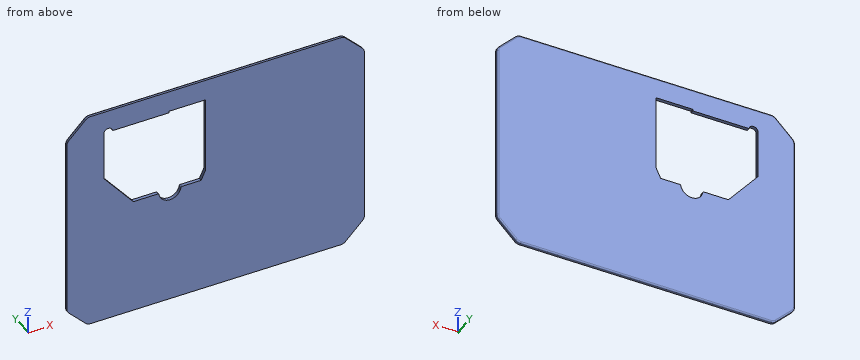
from build123d import *

# Parameters (mm, degrees)
BOSS_EXTRUDE1_DEPTH = 2.5
FILLET2_R           = 5
FILLET3_R           = 1


with BuildPart() as part:
    # Sketch1 → Boss-Extrude1 (new body)
    with BuildSketch(Plane(origin=(0, 0, 0), x_dir=(1, 0, 0), z_dir=(0, 1, 0))):
        Polygon((137.875, 109.125), (-52.875, 109.125), (-68.375, 93.625), (-68.375, -43.375), (-52.875, -58.875), (137.875, -58.875), (153.375, -43.375), (153.375, 93.625), align=None)
        with BuildLine():
            Line((-40.875, -5.193242225), (-18.827366795, 21.125))
            Line((-18.827366795, 21.125), (0.240165454, 21.125))
            ThreePointArc((0.240165454, 21.125), (8.475, 28.875), (16.709834546, 21.125))
            Line((16.709834546, 21.125), (31.683656114, 21.125))
            Line((31.683656114, 21.125), (35.125, 13.735720962))
            Line((35.125, 13.735720962), (35.125, -43.125))
            Line((35.125, -43.125), (7.625, -43.125))
            Line((7.625, -43.125), (7.625, -41.875))
            Line((7.625, -41.875), (-34.162242519, -41.875))
            ThreePointArc((-34.162242519, -41.875), (-37.750692543, -44.740676492), (-40.875, -41.375))
            Line((-40.875, -41.375), (-40.875, -5.193242225))
        make_face(mode=Mode.SUBTRACT)
    extrude(amount=BOSS_EXTRUDE1_DEPTH)

    # Fillet2
    fillet2_edges = [part.edges().sort_by_distance(p)[0] for p in [
        (-68.375, 1.25, 43.375),
        (-68.375, 1.25, -93.625),
        (-52.875, 1.25, -109.125),
        (137.875, 1.25, -109.125),
        (153.375, 1.25, -93.625),
        (153.375, 1.25, 43.375),
        (137.875, 1.25, 58.875),
        (-52.875, 1.25, 58.875),
    ]]
    fillet(fillet2_edges, radius=FILLET2_R)

    # Fillet3
    fillet3_edges = [part.edges().sort_by_distance(p)[0] for p in [
        (16.709834546, 1.25, -21.125),
        (0.240165454, 1.25, -21.125),
        (-68.375, 2.5, -25.125),
        (-60.625, 2.5, -101.375),
        (-60.625, 2.5, 51.125),
        (42.5, 2.5, 58.875),
        (145.625, 2.5, 51.125),
        (153.375, 2.5, -25.125),
        (145.625, 2.5, -101.375),
        (42.5, 2.5, -109.125),
        (-67.994397663, 2.5, 43.21734935),
        (-52.71734935, 2.5, 58.494397663),
        (137.71734935, 2.5, 58.494397663),
        (152.994397663, 2.5, 43.21734935),
        (137.71734935, 2.5, -108.744397663),
        (152.994397663, 2.5, -93.46734935),
        (-52.71734935, 2.5, -108.744397663),
        (-67.994397663, 2.5, -93.46734935),
    ]]
    fillet(fillet3_edges, radius=FILLET3_R)


solid = part.part
The model under review builds one solid part; all positions refer to its coordinate system, in mm. Give positions to 0.01 mm unless a question says otherwise; leave off trailing zeros. Order: outer loops, then holes, each group sorted by start corner. A loop starts at its lowest first (then second) coordinate and runs counter-clockwise, first axis right, second up. Notation, with made-up numbers: M 53,-38 L 71,-38 A27 cw 71,-9 Z; hole C -18.5,-33 d8. An arc over 180 degrees is marked long. Use one line per item in the form item = value. Start each with the question number.
Item 1: To check wall thickness, follow line 1 along Z through (x, y) = (29.5, 0.35) (3 decimals); line 2 along X through (y, z) = (2.1, 28) (3 decimals); line 3 along Z through (x, y) = (-11, 1.3) (3 decimals). State the ranges of each line that lie inside material, in increasing order. Write a range as from..to.
Item 2: We need section A-A on x = 23. Give the boundary of the cut face in (y, z) (3 decimals), plus the area to 3 significant figures.
Item 3: Insertion check: pin 1 Ø1.4 at (y, z) = (1.5, 42.5) entering from +X. The pin has a flat end and moves straight along its axis. Give the tip position at first contact, or say it passes through.
Completed:
q1.line_1 = -109.125..-21.125, 43.125..58.875
q1.line_2 = -68.175..-40.875, 35.125..153.175
q1.line_3 = -109.125..-21.125, 41.875..58.875
q2.outline = M 0,-109.125 L 1.5,-109.125 A1 ccw 2.5,-108.125 L 2.5,-21.125 L 0,-21.125 Z; M 0,43.125 L 2.5,43.125 L 2.5,57.875 A1 ccw 1.5,58.875 L 0,58.875 Z
q2.area = 259 mm²
q3.pin_1 = 153.35
